from build123d import *

# Parameters (mm, degrees)
SKETCH1_W           = 15.875
SKETCH1_H           = 15.875
SKETCH1_R           = 2.34506403
BOSS_EXTRUDE1_DEPTH = 7.9375
SKETCH2_R           = 6.604
CUT_EXTRUDE1_DEPTH  = 3
SKETCH3_R           = 1
CUT_EXTRUDE2_DEPTH  = 1
FILLET1_R           = 0.79375
CIRPATTERN1_COUNT   = 4


with BuildPart() as part:
    # Sketch1 → Boss-Extrude1 (new, symmetric)
    with BuildSketch(Plane(origin=(0, 0, 0), x_dir=(1, 0, 0), z_dir=(0, 1, 0))):
        Rectangle(SKETCH1_W, SKETCH1_H)
        with Locations(Location((0, 0, 0), (0, 0, 270))):
            Circle(SKETCH1_R, mode=Mode.SUBTRACT)
    extrude(amount=BOSS_EXTRUDE1_DEPTH, both=True)

    # Sketch2 → Cut-Extrude1 (cut)
    with BuildSketch(Plane(origin=(0, 7.9375, 0), x_dir=(1, 0, 0), z_dir=(0, 1, 0))):
        with Locations(Location((0, 0, 0), (0, 0, 270))):
            Circle(SKETCH2_R)
    extrude(amount=-CUT_EXTRUDE1_DEPTH, mode=Mode.SUBTRACT)

    # Sketch3 → Cut-Extrude2 (cut)
    with BuildSketch(Plane(origin=(0, 4.9375, 0), x_dir=(1, 0, 0), z_dir=(0, 1, 0))):
        with Locations(Location((-4.7625, 0, 0), (0, 0, 270))):
            Circle(SKETCH3_R)
    cut_extrude2 = extrude(amount=-CUT_EXTRUDE2_DEPTH, mode=Mode.SUBTRACT)

    # Fillet1
    fillet1_edges = [part.edges().sort_by_distance(p)[0] for p in [
        (7.9375, 0, 7.9375),
        (-7.9375, 0, 7.9375),
        (-7.9375, 0, -7.9375),
        (7.9375, 0, -7.9375),
    ]]
    fillet(fillet1_edges, radius=FILLET1_R)

    # CirPattern1: Cut-Extrude2 ×4 about axis
    cirpattern1_axis = Axis((0, 0, 0), (0, 1, 0))
    for i in range(1, CIRPATTERN1_COUNT):
        add(cut_extrude2.rotate(cirpattern1_axis, i * 360 / CIRPATTERN1_COUNT), mode=Mode.SUBTRACT)


solid = part.part
Check sheet for the modelled part. Datum: model origin and axes. Units: mm. A direction names the side the tool comes from. Round coordinates to 2 decimals unless told otherwise and drop trailing zeros. Order: outer loops, then holes, each group sorted by start corner. A loop starts at its lowest first (then second) coordinate and runs counter-clockwise, first axis right, second up.
(1) Cross-section at C-C, the plane x = 0. Enter the section's corners in (y, z), and give its area (3 significant figures).
(2) Go/stop test with flat-tipped pins: P1, Ø6, axis at x = 0, z = 0, coming from the +Y side; P2, Ø1, axis at x = 0, z = -5, coming from the +Y side. Record where each tip stops, or that it passes through.
(3) Access from +Z, -Z, +X, -X, +Y, -Y to the whole of each face (thin tool, end or side, straight path). Record for faces 4 (the flat face through (0, 0, -7.938)), 5 (the cylindrical face through (0.13, 4.44, -3.77)).
(4) Draft check along X on faces 1 (the flat face through (7.938, 0, 0)), 2 (the cylindrical face through (0.7, -1.59, 2.24)), 3 (the flat face through (-2, -7.938, -2)). Enter one of: pulls with the +X half, pulls with the -X half, needs draft (parallel to the pull), parting line crosses it, or undercut.
(5) Cross-section at D-D, the plane y = -2.25. Enter the section's corners in (x, z).
(6) Scan lines: probe 1 along X at (y, z) = (4.25, 0); probe 2 along X at (y, z) = (6.05, 0); probe 3 along Y at (x, z) = (-1.75, -5.25). Record each from-to range of solid material in increasing order.
(7) Cross-section at B-B, the plane y = 6.5. Enter the section's corners in (x, z), and give its area (3 significant figures).
(8) Cross-section at A-A, the plane z = 0. Enter the section's corners in (x, y), and give its area (3 significant figures).
Check sheet entries:
1. outline: (-7.94, -7.94) - (7.94, -7.94) - (7.94, -6.6) - (4.94, -6.6) - (4.94, -5.76) - (3.94, -5.76) - (3.94, -3.76) - (4.94, -3.76) - (4.94, -2.35) - (-7.94, -2.35) - close; (-7.94, 2.35) - (4.94, 2.35) - (4.94, 3.76) - (3.94, 3.76) - (3.94, 5.76) - (4.94, 5.76) - (4.94, 6.6) - (7.94, 6.6) - (7.94, 7.94) - (-7.94, 7.94) - close
1. area: 148 mm2
2. P1: stops at y = 4.94
2. P2: stops at y = 3.94
3. face 4: -Z, +X, -X, +Y, -Y
3. face 5: +Y
4. face 1: pulls with the +X half
4. face 2: undercut
4. face 3: needs draft
5. outline: (-7.94, -7.14) arc R0.79 ccw to (-7.14, -7.94) - (7.14, -7.94) arc R0.79 ccw to (7.94, -7.14) - (7.94, 7.14) arc R0.79 ccw to (7.14, 7.94) - (-7.14, 7.94) arc R0.79 ccw to (-7.94, 7.14) - close; hole circle Ø4.69 at (0, 0)
6. probe 1: x = -7.94 to -5.76, -3.76 to -2.35, 2.35 to 3.76, 5.76 to 7.94
6. probe 2: x = -7.94 to -6.6, 6.6 to 7.94
6. probe 3: y = -7.94 to 4.94
7. outline: (-7.94, -7.14) arc R0.79 ccw to (-7.14, -7.94) - (7.14, -7.94) arc R0.79 ccw to (7.94, -7.14) - (7.94, 7.14) arc R0.79 ccw to (7.14, 7.94) - (-7.14, 7.94) arc R0.79 ccw to (-7.94, 7.14) - close; hole circle Ø13.21 at (0, 0)
7. area: 114 mm2
8. outline: (-7.94, -7.94) - (-2.35, -7.94) - (-2.35, 4.94) - (-3.76, 4.94) - (-3.76, 3.94) - (-5.76, 3.94) - (-5.76, 4.94) - (-6.6, 4.94) - (-6.6, 7.94) - (-7.94, 7.94) - close; (2.35, -7.94) - (7.94, -7.94) - (7.94, 7.94) - (6.6, 7.94) - (6.6, 4.94) - (5.76, 4.94) - (5.76, 3.94) - (3.76, 3.94) - (3.76, 4.94) - (2.35, 4.94) - close
8. area: 148 mm2
